The listing builds one solid part. Answer for the finished solid, in the listing's coordinates (mm). A direction names the side the tool comes from. Give positions to 0.01 mm unless a question says otherwise; leave off trailing zeros. Write each loop counter-clockwise with the first axis right and the second up, starting at its lowest first coordinate (ties: lowest second). Pieces come first, ordered by that corner, then holes.
```python
from build123d import *

# Parameters (mm, degrees)
SKETCH_1_W             = 166
SKETCH_1_H             = 108
EXTRUDE_1_DEPTH        = 10
SKETCH_2_R             = 2
CUT_EXTRUDE_834_DEPTH  = 11
SKETCH_4_W             = 128
SKETCH_4_H             = 96
CUT_EXTRUDE_1103_DEPTH = 11
SKETCH_5_W             = 17.5
SKETCH_5_H             = 13
USB_DEPTH              = 11
FILLET_1_R             = 3
CHAMFER_1_SIZE         = 3
FILLET_2_R             = 3


with BuildPart() as part:
    # Эскиз1 → Бобышка-Вытянуть1 (new body)
    with BuildSketch(Plane(origin=(0, 0, 0), x_dir=(1, 0, 0), z_dir=(0, 1, 0))):
        Rectangle(SKETCH_1_W, SKETCH_1_H)
    extrude(amount=EXTRUDE_1_DEPTH)

    # Эскиз2 → Cut-Extrude 834 (cut, through all)
    with BuildSketch(Plane(origin=(0, 10, 0), x_dir=(1, 0, 0), z_dir=(0, 1, 0))):
        with Locations((-73, 44)):
            Circle(SKETCH_2_R)
        with Locations((73, 44)):
            Circle(SKETCH_2_R)
        with Locations((-73, -44)):
            Circle(SKETCH_2_R)
        with Locations((73, -44)):
            Circle(SKETCH_2_R)
    extrude(amount=-CUT_EXTRUDE_834_DEPTH, mode=Mode.SUBTRACT)

    # Эскиз4 → Cut-Extrude 1103 (cut, through all)
    with BuildSketch(Plane(origin=(0, 10, 0), x_dir=(1, 0, 0), z_dir=(0, 1, 0))):
        with Locations((1.5, 0)):
            Rectangle(SKETCH_4_W, SKETCH_4_H)
    extrude(amount=-CUT_EXTRUDE_1103_DEPTH, mode=Mode.SUBTRACT)

    # Эскиз5 → usb (cut, through all)
    with BuildSketch(Plane(origin=(0, 10, 0), x_dir=(1, 0, 0), z_dir=(0, 1, 0))):
        with Locations((74.25, 32.1)):
            Rectangle(SKETCH_5_W, SKETCH_5_H)
    extrude(amount=-USB_DEPTH, mode=Mode.SUBTRACT)

    # Скругление1
    fillet_1_edges = [part.edges().sort_by_distance(p)[0] for p in [
        (65.5, 5, -48),
        (65.5, 5, 48),
        (-62.5, 5, 48),
        (-62.5, 5, -48),
    ]]
    fillet(fillet_1_edges, radius=FILLET_1_R)

    # Фаска1
    chamfer_1_edges = [part.edges().sort_by_distance(p)[0] for p in [
        (83, 5, -38.6),
        (83, 5, -25.6),
    ]]
    chamfer(chamfer_1_edges, length=CHAMFER_1_SIZE)

    # Скругление2
    fillet_2_edges = [part.edges().sort_by_distance(p)[0] for p in [
        (65.5, 5, -25.6),
        (65.5, 5, -38.6),
    ]]
    fillet(fillet_2_edges, radius=FILLET_2_R)


solid = part.part
```
Item 1: A cutting plane is placed at A-A, the plane x = -73. Give the vertices of the cut face in (y, z), plus the area to 3 significant figures.
Conclusion:
outline: (0, -54) - (10, -54) - (10, -46) - (0, -46) - close; (0, -42) - (10, -42) - (10, 42) - (0, 42) - close; (0, 46) - (10, 46) - (10, 54) - (0, 54) - close
area: 1,000 mm2
Item 2: Determine the mould class of faces 4 (the face through (65.5, 5, -43)), 5 (the face through (-1, 5, 54)), 6 (the face through (-0.4, 10, -48.3)) for opening direction Z: pulls with the +Z half, pulls with the -Z half, needs draft (parallel to the pull), parting line crosses it, or undercut.
Conclusion:
face 4: undercut
face 5: pulls with the +Z half
face 6: needs draft
Item 3: Consider probe 1 along X at (y, z) = (6, -44); probe 2 along Z at (x, y) = (73, 6.5); probe 3 along Z at (x, y) = (48, 8). Determine where each line is inside the solid, lowest interval first.
Conclusion:
probe 1: x = -83 to -75, -71 to -62.5, 65.5 to 71, 75 to 83
probe 2: z = -54 to -46, -42 to -38.6, -25.6 to 42, 46 to 54
probe 3: z = -54 to -48, 48 to 54
Item 4: A cutting plane is placed at C-C, the plane x = -18. Give the vertices of the cut face in (y, z).
Conclusion:
outline: (0, -54) - (10, -54) - (10, -48) - (0, -48) - close; (0, 48) - (10, 48) - (10, 54) - (0, 54) - close
Item 5: A cutting plane is placed at D-D, the plane y = 2.25. Give the vertices of the cut face in (x, z), plus the area to 3 significant figures.
Conclusion:
outline: (-83, -54) - (83, -54) - (83, -41.6) - (80, -38.6) - (68.5, -38.6) arc R3 ccw to (65.5, -41.6) - (65.5, -45) arc R3 cw to (62.5, -48) - (-59.5, -48) arc R3 cw to (-62.5, -45) - (-62.5, 45) arc R3 cw to (-59.5, 48) - (62.5, 48) arc R3 cw to (65.5, 45) - (65.5, -22.6) arc R3 ccw to (68.5, -25.6) - (80, -25.6) - (83, -22.6) - (83, 54) - (-83, 54) - close; hole circle Ø4 at (-73, -44); hole circle Ø4 at (-73, 44); hole circle Ø4 at (73, -44); hole circle Ø4 at (73, 44)
area: 5,360 mm2
Item 6: Which of the six approach directions +Z, -Z, +X, -X, +Y, -Y give full straight-line access (tool end or side, diameter ignored) to faces 1 (the face through (64.64, 4.93, -47.1)), 2 (the face through (74, 5, -25.6)), 3 (the face through (-1, 5, -54))?
Conclusion:
face 1: +Y, -Y
face 2: +X, +Y, -Y
face 3: -Z, +X, -X, +Y, -Y
Item 7: A cutting plane is placed at B-B, the plane z = -11. Give the vertices of the cut face in (x, y).
Conclusion:
outline: (-83, 0) - (-62.5, 0) - (-62.5, 10) - (-83, 10) - close; (65.5, 0) - (83, 0) - (83, 10) - (65.5, 10) - close
